Geometry: final body of the model. Coordinates: model frame, mm. Give positions to 0.01 mm unless a question says otherwise; leave off trailing zeros. Order: outer loops, then holes, each group sorted by start corner. A loop starts at its lowest first (then second) coordinate and runs counter-clockwise, first axis right, second up. Notation, with made-up numbers: (-2.75, 59.5) -> (10.25, 59.5) arc R18 cw to (10.25, 91.5) -> close; hole circle Ø10 at (-27, 63). An arc over 180 degrees is marked (long way). One line per question, with ' | ' between items.
from build123d import *

# Parameters (mm, degrees)
SKETCH_W    = 200
SKETCH_H    = 100
SKETCH_R    = 30
SKETCH_R_2  = 10
PAD_DEPTH   = 10
FILLET_R    = 10
FILLET001_R = 10


with BuildPart() as part:
    # Sketch → Pad (new body)
    with BuildSketch(Plane.XZ):
        Rectangle(SKETCH_W, SKETCH_H)
        Circle(SKETCH_R, mode=Mode.SUBTRACT)
        with Locations((-70, 20)):
            Circle(SKETCH_R_2, mode=Mode.SUBTRACT)
        with Locations((70, 20)):
            Circle(SKETCH_R_2, mode=Mode.SUBTRACT)
        with Locations((70, -20)):
            Circle(SKETCH_R_2, mode=Mode.SUBTRACT)
        with Locations((-70, -20)):
            Circle(SKETCH_R_2, mode=Mode.SUBTRACT)
    extrude(amount=PAD_DEPTH)

    # Fillet
    fillet_edges = [part.edges().sort_by_distance(p)[0] for p in [
        (100, -5, -50),
        (100, -5, 50),
        (-100, -5, 50),
    ]]
    fillet(fillet_edges, radius=FILLET_R)

    # Fillet001
    fillet001_edges = [part.edges().sort_by_distance(p)[0] for p in [
        (-100, -5, -50),
    ]]
    fillet(fillet001_edges, radius=FILLET001_R)


solid = part.part
1) Material intervals for probe 1 along Z at (x, y) = (70, -7.5); probe 2 along X at (y, z) = (-4, -26.5); probe 3 along Z at (x, y) = (-71, -1.75), sorted ascending. Write a range as from..to.
Check result:
probe 1: z = -50..-30, -10..10, 30..50 | probe 2: x = -100..-77.6, -62.4..-14.06, 14.06..62.4, 77.6..100 | probe 3: z = -50..-29.95, -10.05..10.05, 29.95..50
2) Section D-D on x = 0. Return loops of the section in (y, z).
Check result:
outline: (-10, -50) -> (0, -50) -> (0, -30) -> (-10, -30) -> close; (-10, 30) -> (0, 30) -> (0, 50) -> (-10, 50) -> close
3) Section C-C on z = 20. Return loops of the section in (x, y), plus the area to 3 significant figures.
Check result:
outline: (-100, -10) -> (-80, -10) -> (-80, 0) -> (-100, 0) -> close; (-60, -10) -> (-22.36, -10) -> (-22.36, 0) -> (-60, 0) -> close; (22.36, -10) -> (60, -10) -> (60, 0) -> (22.36, 0) -> close; (80, -10) -> (100, -10) -> (100, 0) -> (80, 0) -> close | area: 1,150 mm^2
4) Section B-B on x = -70. Return loops of the section in (y, z).
Check result:
outline: (-10, -50) -> (0, -50) -> (0, -30) -> (-10, -30) -> close; (-10, -10) -> (0, -10) -> (0, 10) -> (-10, 10) -> close; (-10, 30) -> (0, 30) -> (0, 50) -> (-10, 50) -> close
5) Section A-A on y = -2.5. Return loops of the section in (x, z).
Check result:
outline: (-100, -40) arc R10 ccw to (-90, -50) -> (90, -50) arc R10 ccw to (100, -40) -> (100, 40) arc R10 ccw to (90, 50) -> (-90, 50) arc R10 ccw to (-100, 40) -> close; hole circle Ø20 at (-70, -20); hole circle Ø20 at (-70, 20); hole circle Ø60 at (0, 0); hole circle Ø20 at (70, -20); hole circle Ø20 at (70, 20)
6) Pull-direction query (Z, two-part tool) for faces 1 (the flat face through (21, 0, 23)), 2 (the cylindrical face through (60, -5, -20)), 3 (the flat face through (-1, -5, 50)); classes: +Z half, -Z half, draft (parallel to the pull), parting line (faces both ways), or undercut.
Check result:
face 1: draft | face 2: undercut | face 3: +Z half
